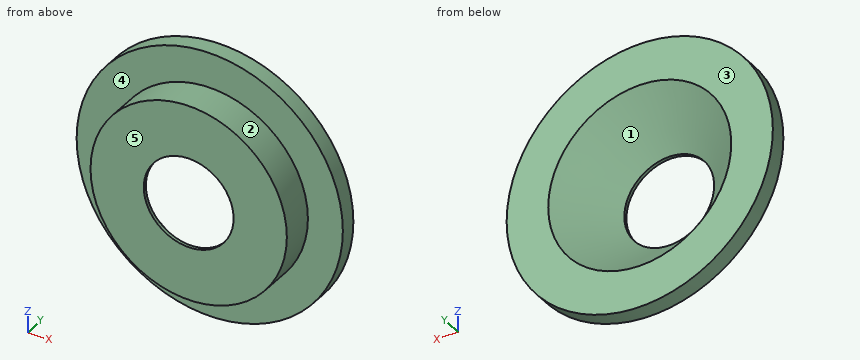
from build123d import *

# Parameters (mm, degrees)
SKETCH1_R           = 2.95
BOSS_EXTRUDE1_DEPTH = 1
SKETCH2_R           = 4
BOSS_EXTRUDE2_DEPTH = 0.5


with BuildPart() as part:
    # Sketch1 → Boss-Extrude1 (new body)
    with BuildSketch(Plane(origin=(0, 0, 0), x_dir=(1, 0, 0), z_dir=(0, 1, 0))):
        Circle(SKETCH1_R)
    extrude(amount=BOSS_EXTRUDE1_DEPTH)

    # Sketch2 → Boss-Extrude2 (add)
    with BuildSketch(Plane(origin=(0, 1, 0), x_dir=(1, 0, 0), z_dir=(0, 1, 0))):
        Circle(SKETCH2_R)
    extrude(amount=BOSS_EXTRUDE2_DEPTH)

    # Sketch3 → CSK for M2.5 Flat Head Machine Screw1 (revolve, cut)
    with BuildSketch(Plane(origin=(0, 1.5, 0), x_dir=(0, 0, 1), z_dir=(1, 0, 0))):
        Polygon((0, 0), (0, 2.311161836), (1.35, 1.5), (1.35, 1.4), (2.75, 0), align=None)
    revolve(axis=Axis((0, 7.85, 0), (0, -1, 0)), mode=Mode.SUBTRACT)


solid = part.part
Input: part model. Units: mm. Frame: model coordinates. Face numbers are marked on the shaded views. A direction names the side the tool comes from. Give positions to 0.01 mm unless a question says otherwise; leave off trailing zeros. Order: outer loops, then holes, each group sorted by start corner. A loop starts at its lowest first (then second) coordinate and runs counter-clockwise, first axis right, second up. Notation, with made-up numbers: M 87.5,43 L 126.5,43 A15 cw 126.5,49 Z; hole C 81.25,-38 d9. An arc over 180 degrees is marked long. Answer as a JSON object with one key per item and string values.
1. Cut plane A-A, the plane x = 0. Output: boundary loops of the cut face in (y, z), and give its area (3 significant figures).
Result sheet:
{"outline": "M 0,-2.95 L 1,-2.95 L 1,-4 L 1.5,-4 L 1.5,-2.75 L 0.1,-1.35 L 0,-1.35 Z; M 0,1.35 L 0.1,1.35 L 1.5,2.75 L 1.5,4 L 1,4 L 1,2.95 L 0,2.95 Z", "area": "3.89 mm²"}
2. Reachability of the marked faces 4 and 5 from +Z, -Z, +X, -X, +Y, -Y: full face, straight path, thin tool, end or side. Return the list, or none.
Result sheet:
{"face 4": "-Y", "face 5": "+Z, -Z, +X, -X, -Y"}
3. Cut plane C-C, the plane y = 1.3. Output: boundary loops of the cut face in (x, z).
Result sheet:
{"outline": "C 0,0 d8; hole C 0,0 d5.1"}
4. Ray query, line 1 (Z direction, x = 0, y = 0.05); line 2 (Y direction, x = 3.25, z = -0.5); line 3 (X direction, y = 0.7, z = 1.5). Return the intervals inside material, ascending. Write a range as [from, to].
Result sheet:
{"line 1": "[-2.95, -1.35], [1.35, 2.95]", "line 2": "[1, 1.5]", "line 3": "[-2.54, -1.25], [1.25, 2.54]"}
5. Cut plane D-D, the plane y = 0.9. Output: boundary loops of the cut face in (x, z).
Result sheet:
{"outline": "C 0,0 d5.9; hole C 0,0 d4.3"}
6. Pull-direction query (X, two-part tool) for the marked faces 1, 2 and 3; classes: +X half, -X half, draft (parallel to the pull), parting line (faces both ways), or undercut.
Result sheet:
{"face 1": "undercut", "face 2": "parting line", "face 3": "draft"}
7. Cut plane B-B, the plane z = 0. Output: boundary loops of the cut face in (x, y).
Result sheet:
{"outline": "M -4,1 L -2.95,1 L -2.95,0 L -1.35,0 L -1.35,0.1 L -2.75,1.5 L -4,1.5 Z; M 1.35,0 L 2.95,0 L 2.95,1 L 4,1 L 4,1.5 L 2.75,1.5 L 1.35,0.1 Z"}
